Autodesk Inventor part; units mm, degrees
ref_plane "YZ Plane" through (0, 0, 0) normal (1, 0, 0) x (0, 1, 0)
ref_plane "XZ Plane" through (0, 0, 0) normal (0, 1, 0) x (-1, 0, 0)
ref_plane "XY Plane" through (0, 0, 0) normal (0, 0, 1) x (1, 0, 0)
sketch "Sketch1" plane through (0, 0, 0) normal (0, 0, 1) x (1, 0, 0)
  line L0 (-27.45, -52.45) -> (27.45, -52.45)
  line L1 (52.45, -27.45) -> (52.45, 27.45)
  line L2 (27.45, 52.45) -> (-27.45, 52.45)
  line L3 (-52.45, 27.45) -> (-52.45, -27.45)
  line L4 (-52.45, -52.45) -> (52.45, 52.45) construction
  line L5 (52.45, -52.45) -> (-52.45, 52.45) construction
  arc A0 (-27.45, 52.45) -> (-52.45, 27.45) centre (-27.45, 27.45) ccw
  arc A1 (-52.45, -27.45) -> (-27.45, -52.45) centre (-27.45, -27.45) ccw
  arc A2 (27.45, -52.45) -> (52.45, -27.45) centre (27.45, -27.45) ccw
  arc A3 (52.45, 27.45) -> (27.45, 52.45) centre (27.45, 27.45) ccw
  line L6 (-35, 35) -> (35, 35) construction
  line L7 (35, 35) -> (35, -35) construction
  line L8 (35, -35) -> (-35, -35) construction
  line L9 (-35, -35) -> (-35, 35) construction
  line L10 (-35, 35) -> (35, -35) construction
  line L11 (35, 35) -> (-35, -35) construction
  circle A4 centre (35, 35) radius 1.55
  circle A5 centre (35, -35) radius 1.55
  circle A6 centre (-35, -35) radius 1.55
  circle A7 centre (-35, 35) radius 1.55
  point P0 (0, 0)
  dimension "d0" = 104.9
  dimension "d1" = 104.9
  dimension "d2" = 25
  dimension "d6" = 70
  dimension "d7" = 3.1
extrude "Extrusion1" add sketch "Sketch1" along normal blind 2.5
equation "\"d1\" = d0"
properties part number "NewFront_D"
Could you check a few things on this model? Use its own coordinates, in mm. Give positions to 0.01 mm unless a question says otherwise; leave off trailing zeros. Write each loop counter-clockwise with the first axis right and the second up, starting at its lowest first coordinate (ties: lowest second). Pieces come first, ordered by that corner, then holes. Notation, with made-up numbers: (42, -14) - (76, -14) arc R20 cw to (76, 10) - close; hole circle Ø9 at (70, 43.25). An arc over 180 degrees is marked (long way). Use CSV: the item, a comma, the result in double quotes. Start each with the question number.
Item 1: If I drill on line 1 along Y through (x, z) = (35, 1.3); line 2 along Y through (x, z) = (41, 2.1); line 3 along X through (y, z) = (29, 0.55), over which ranges is the centre line in solid material (lowest first)?
Item 2: I want a section at D-D, the plane x = -39. Please give me the cut outline in (y, z).
Item 3: I'm going to push flat-ended pins straight in: pin 1 (4 mm diameter, centred on x = -35, y = -35, fed in from -Z); pin 2 (2.5 mm diameter, centred on x = 35, y = -35, fed in from +Z). Where does each tip first touch, or does it pass through?
Item 4: I want a section at B-B, the plane x = 35. Please give me the cut outline in (y, z), then the cut area to 3 significant figures.
Item 5: If we mould it in two halves opening along Y, with no side actions, what happens to faces 1 (the face through (-33.522, 34.534, 1.232)), 2 (the face through (-45.321, 44.932, 1.232)), 3 (the face through (36.478, 34.534, 1.232)), 4 (the face through (52.45, 0, 1))? For each: pulls with the +Y half, pulls with the -Y half, needs draft (parallel to the pull), parting line crosses it, or undercut.
Item 6: I want a section at A-A, the plane z = 1.35. Please give me the cut outline in (x, y).
Findings:
1,line 1,"y = -51.28 to -36.55, -33.45 to 33.45, 36.55 to 51.28"
1,line 2,"y = -48.46 to 48.46"
1,line 3,"x = -52.4 to 52.4"
2,outline,"(-49.62, 0) - (49.62, 0) - (49.62, 2.5) - (-49.62, 2.5) - close"
3,pin 1,"stops at z = 0"
3,pin 2,"passes through"
4,outline,"(-51.28, 0) - (-36.55, 0) - (-36.55, 2.5) - (-51.28, 2.5) - close; (-33.45, 0) - (33.45, 0) - (33.45, 2.5) - (-33.45, 2.5) - close; (36.55, 0) - (51.28, 0) - (51.28, 2.5) - (36.55, 2.5) - close"
4,area,"241 mm2"
5,face 1,"undercut"
5,face 2,"pulls with the +Y half"
5,face 3,"undercut"
5,face 4,"needs draft"
6,outline,"(-52.45, -27.45) arc R25 ccw to (-27.45, -52.45) - (27.45, -52.45) arc R25 ccw to (52.45, -27.45) - (52.45, 27.45) arc R25 ccw to (27.45, 52.45) - (-27.45, 52.45) arc R25 ccw to (-52.45, 27.45) - close; hole circle Ø3.1 at (-35, -35); hole circle Ø3.1 at (-35, 35); hole circle Ø3.1 at (35, -35); hole circle Ø3.1 at (35, 35)"
